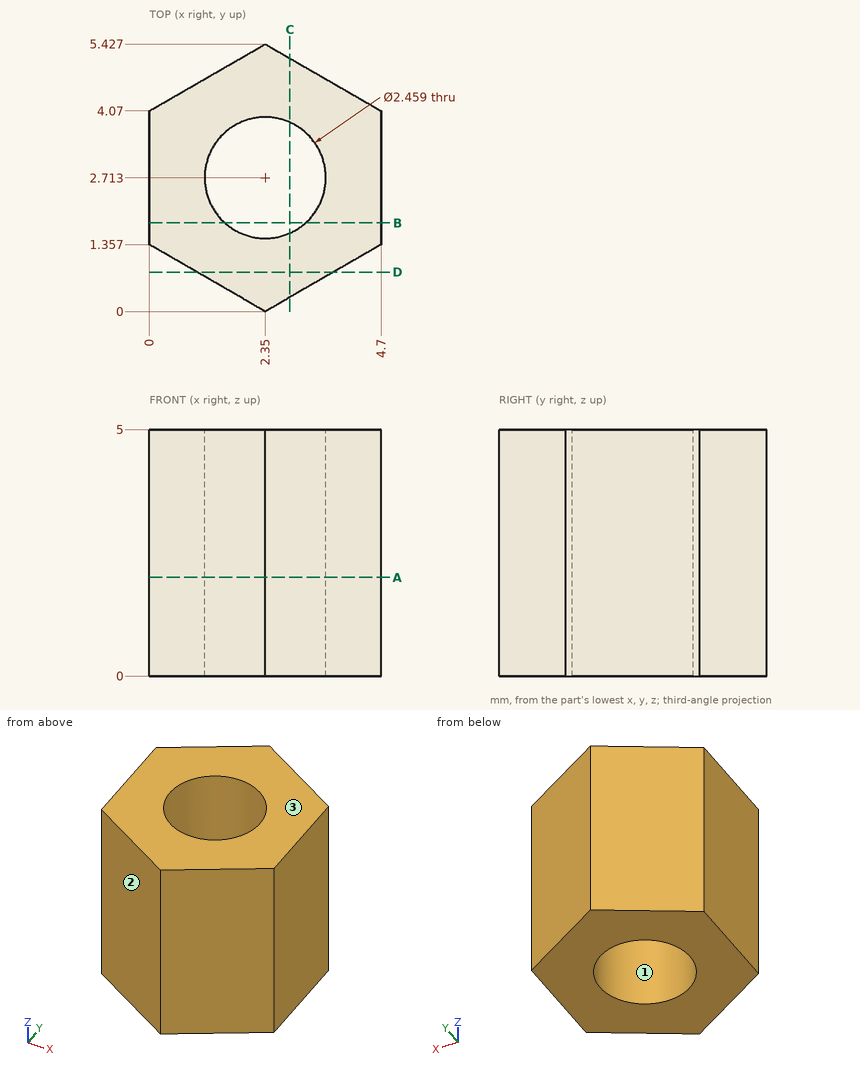
Design review of the part shown in the three views and the two pictorial views. Dimensions are in mm from the part's minimum x, y and z. Give positions to 0.01 mm unless a question says otherwise; leave off trailing zeros. Loops run counter-clockwise (first coordinate to the right, second up) from the corner with the lowest first, then second, coordinate; pieces in that order, holes last. Notation, with made-up numbers: (-36, 4.5) -> (-14, 4.5) arc R11 ccw to (-14, 17.5) -> close; hole circle Ø8 at (10.5, 26). An arc over 180 degrees is marked (long way). Put each result on its own line as item: value. Start each with the question number.
1. Wall thickness on probe 1 along Y at (x, z) = (1.55, 4.75) (1 decimal); probe 2 along X at (y, z) = (2.6, 0.65) (1 decimal); probe 3 along Y at (x, z) = (3.1, 3.45) (1 decimal): over which ranges is each line inside the solid? List them lowest first.
2. We need section D-D on y = 0.8. State the section outline as (x, z) points (1 decimal).
3. Clearance check with flat-ended pins moving along their axes: P1, Ø2, axis at x = 4, z = 0.5, coming from the -Y side (1 decimal); P2, Ø1.5, axis at x = 2.35, y = 2.71, coming from the +Z side. State where each tip first meets the part, or that it passes through.
4. We need section B-B on y = 1.8. State the section outline as (x, z) points.
5. Mouldability with a two-part tool opening along Y and no side actions: class the marked faces 1, 2 and 3 as released by +Y, released by -Y, zero draft, split by the parting line, or undercut.
6. We need section A-A on z = 2. State the section outline as (x, y) points.
7. We need section C-C on x = 2.85. State the section outline as (y, z) points.
Determined:
1. probe 1: 0.5 to 1.8, 3.6 to 5
1. probe 2: 0 to 1.1, 3.6 to 4.7
1. probe 3: 0.4 to 1.7, 3.7 to 5
2. outline: (1, 0) -> (3.7, 0) -> (3.7, 5) -> (1, 5) -> close
3. P1: y = 0.4
3. P2: through
4. outline: (0, 0) -> (1.53, 0) -> (1.53, 5) -> (0, 5) -> close; (3.17, 0) -> (4.7, 0) -> (4.7, 5) -> (3.17, 5) -> close
5. face 1: undercut
5. face 2: released by -Y
5. face 3: zero draft
6. outline: (0, 1.36) -> (2.35, 0) -> (4.7, 1.36) -> (4.7, 4.07) -> (2.35, 5.43) -> (0, 4.07) -> close; hole circle Ø2.46 at (2.35, 2.71)
7. outline: (0.29, 0) -> (1.59, 0) -> (1.59, 5) -> (0.29, 5) -> close; (3.84, 0) -> (5.14, 0) -> (5.14, 5) -> (3.84, 5) -> close
